Source: CAD feature listing. Evaluate the final solid. Frame: model axes, mm. A direction names the side the tool comes from. Give positions to 0.01 mm unless a question says otherwise; leave off trailing zeros. Write each loop counter-clockwise with the first axis right and the second up, starting at its lowest first coordinate (ties: lowest second). Pieces come first, ordered by that corner, then holes. Notation, with made-up numbers: M 39.5,47 L 60.5,47 A29 cw 60.5,67 Z; hole C -11.75,72 d7. An arc over 180 degrees is marked long. Use CSV: the item, a comma, the result in double quotes. Start each with the question number.
from build123d import *

# Parameters (mm, degrees)
SKETCH1_W               = 15.875
SKETCH1_H               = 15.875
BOSS_EXTRUDE1_DEPTH     = 149.225
CUT_EXTRUDE1_DEPTH      = 151.276811772
CUT_EXTRUDE1_DEPTH_BACK = 151.276811772
CUT_EXTRUDE2_START      = -1.5875
SKETCH4_W               = 12.7
SKETCH4_H               = 14.2875
CUT_EXTRUDE2_DEPTH      = 149.225
CUT_EXTRUDE4_DEPTH      = 151.276811772
SKETCH6_W               = 6.35
SKETCH6_H               = 1.5875
CUT_EXTRUDE5_DEPTH      = 1.5875
SKETCH7_W               = 1.5875
SKETCH7_H               = 0.910155424
CUT_EXTRUDE6_DEPTH      = 1.5875
SKETCH8_R               = 1.5875
SKETCH8_W               = 1.5875
SKETCH8_H               = 3.96875
CUT_EXTRUDE7_DEPTH      = 151.276811772
SKETCH9_R               = 3.175
CUT_EXTRUDE8_DEPTH      = 151.276811772
BOSS_EXTRUDE2_START     = 0.396875
SKETCH10_R              = 1.5875
BOSS_EXTRUDE2_DEPTH     = 0.396875
SKETCH11_W              = 12.7
SKETCH11_H              = 14.601302857
CUT_EXTRUDE9_DEPTH      = 2.54


with BuildPart() as part:
    # Sketch1 → Boss-Extrude1 (new body)
    with BuildSketch(Plane.XY):
        Rectangle(SKETCH1_W, SKETCH1_H)
    extrude(amount=-BOSS_EXTRUDE1_DEPTH)

    # Sketch2 → Cut-Extrude1 (cut, two sides: drawn at the far end of the back side and taken through both)
    with BuildSketch(Plane(origin=(7.9375, 0, 0), x_dir=(0, 0, -1), z_dir=(1, 0, 0)).offset(-CUT_EXTRUDE1_DEPTH_BACK)):
        with BuildLine():
            Line((149.225, 7.9375), (12.7, 7.9375))
            Line((12.7, 7.9375), (31.483553311, 4.7625))
            Line((31.483553311, 4.7625), (109.68727062, 4.7625))
            Line((109.68727062, 4.7625), (112.817862839, 5.291666667))
            Line((112.817862839, 5.291666667), (119.167862839, 5.291666667))
            Line((119.167862839, 5.291666667), (122.298455057, 4.7625))
            Line((122.298455057, 4.7625), (133.410955057, 4.7625))
            Line((133.410955057, 4.7625), (145.71107606, 1.420918197))
            ThreePointArc((145.71107606, 1.420918197), (148.245868191, -0.282331443), (149.225, -3.175))
            Line((149.225, -3.175), (149.225, 7.9375))
        make_face()
        with BuildLine():
            Line((149.225, -7.9375), (149.225, -3.175))
            ThreePointArc((149.225, -3.175), (147.830096045, -6.542596045), (144.4625, -7.9375))
            Line((144.4625, -7.9375), (149.225, -7.9375))
        make_face()
    extrude(amount=CUT_EXTRUDE1_DEPTH + CUT_EXTRUDE1_DEPTH_BACK, mode=Mode.SUBTRACT)

    # Sketch4 → Cut-Extrude2 (cut)
    with BuildSketch(Plane.XY.offset(CUT_EXTRUDE2_START)):
        with Locations((0, 0.79375)):
            Rectangle(SKETCH4_W, SKETCH4_H)
    extrude(amount=-CUT_EXTRUDE2_DEPTH, mode=Mode.SUBTRACT)

    # Sketch5 → Cut-Extrude4 (cut, through all)
    with BuildSketch(Plane.XZ.offset(7.9375)):
        Polygon((2.38125, -6.35), (-2.38125, -6.35), (-4.283584011, -2.497655424), (-6.35, -2.497655424), (-6.35, -1.5875), (-0.79375, -1.5875), (-0.79375, 0), (0.79375, 0), (0.79375, -1.5875), (6.35, -1.5875), (6.35, -2.497655424), (4.283584011, -2.497655424), align=None)
    extrude(amount=-CUT_EXTRUDE4_DEPTH, mode=Mode.SUBTRACT)

    # Sketch6 → Cut-Extrude5 (cut)
    with BuildSketch(Plane.XY):
        Polygon((0.79375, 4.7625), (2.38125, 4.7625), (4.7625, 7.9375), (0.79375, 7.9375), align=None)
        Polygon((-0.79375, 4.7625), (-2.38125, 4.7625), (-4.7625, 7.9375), (-0.79375, 7.9375), align=None)
        with Locations((0, -7.14375)):
            Rectangle(SKETCH6_W, SKETCH6_H)
    extrude(amount=-CUT_EXTRUDE5_DEPTH, mode=Mode.SUBTRACT)

    # Sketch7 → Cut-Extrude6 (cut)
    with BuildSketch(Plane.XZ.offset(7.9375)):
        with Locations((7.14375, -2.042577712)):
            Rectangle(SKETCH7_W, SKETCH7_H)
        with Locations((-7.14375, -2.042577712)):
            Rectangle(SKETCH7_W, SKETCH7_H)
    extrude(amount=-CUT_EXTRUDE6_DEPTH, mode=Mode.SUBTRACT)

    # Sketch8 → Cut-Extrude7 (cut, through all)
    with BuildSketch(Plane(origin=(7.9375, 0, 0), x_dir=(0, 0, -1), z_dir=(1, 0, 0))):
        with Locations((144.4625, -3.175)):
            Circle(SKETCH8_R)
        with Locations((2.38125, -1.190625)):
            Rectangle(SKETCH8_W, SKETCH8_H)
        with BuildLine():
            Line((7.14375, -3.175), (10.31875, -3.175))
            ThreePointArc((10.31875, -3.175), (11.1125, -3.96875), (10.31875, -4.7625))
            Line((10.31875, -4.7625), (7.14375, -4.7625))
            ThreePointArc((7.14375, -4.7625), (6.35, -3.96875), (7.14375, -3.175))
        make_face()
    extrude(amount=-CUT_EXTRUDE7_DEPTH, mode=Mode.SUBTRACT)

    # Sketch9 → Cut-Extrude8 (cut, through all)
    with BuildSketch(Plane.XZ.offset(7.9375)):
        with Locations(Location((0, -22.225, 0), (0, 0, 270))):
            Circle(SKETCH9_R)
        with Locations(Location((0, -122.2375, 0), (0, 0, 270))):
            Circle(SKETCH9_R)
    extrude(amount=-CUT_EXTRUDE8_DEPTH, mode=Mode.SUBTRACT)

    # Sketch10 → Boss-Extrude2 (add)
    with BuildSketch(Plane(origin=(7.9375, 0, 0), x_dir=(0, 0, -1), z_dir=(1, 0, 0)).offset(BOSS_EXTRUDE2_START)):
        with BuildLine():
            Line((144.4625, 0), (19.05, 0))
            ThreePointArc((19.05, 0), (18.25625, -0.79375), (19.05, -1.5875))
            Line((19.05, -1.5875), (141.712869343, -1.5875))
            ThreePointArc((141.712869343, -1.5875), (146.05, -5.924630657), (144.4625, 0))
        make_face()
        with Locations((144.4625, -3.175)):
            Circle(SKETCH10_R, mode=Mode.SUBTRACT)
    boss_extrude2 = extrude(amount=-BOSS_EXTRUDE2_DEPTH)

    # Mirror1: Boss-Extrude2 across plane
    add(boss_extrude2.mirror(Plane(origin=(0, 0, 0), x_dir=(0, 0, 1), z_dir=(1, 0, 0))))

    # Sketch11 → Cut-Extrude9 (cut)
    with BuildSketch(Plane(origin=(0, -6.35, 0), x_dir=(1, 0, 0), z_dir=(0, 1, 0))):
        with Locations((0, 140.711606485)):
            Rectangle(SKETCH11_W, SKETCH11_H)
    extrude(amount=-CUT_EXTRUDE9_DEPTH, mode=Mode.SUBTRACT)


solid = part.part
1. First-contact query: pin 1 (8 mm diameter, centred on x = -2, z = -58, fed in from +Y); pin 2 (3 mm diameter, centred on x = 6.5, y = 2.5, fed in from -Z); pin 3 (0.8 mm diameter, centred on y = -3, z = -1, fed in from -X); pin 4 (4 mm diameter, centred on x = 0, z = -122.24, fed in from -Y). Flat tips, straight axial feed; report the tip coordinate or a pass-through.
2. Access query for faces 1 (the flat face through (-6.35, 0, -74)), 2 (the flat face through (-3.555, 6.328, -0.783)), 3 (the cylindrical face through (0.954, -7.155, -25.253)). Directions: +Z, -Z, +X, -X, +Y, -Y. A direction counts if a zero-diameter tool reaches every point of the face in a straight line with its end or side. Return the directions, or none.
3. Pull-direction query (Z, two-part tool) for faces 4 (the flat face through (8.334, -1, -83)), 5 (the cylindrical face through (0.954, -7.155, -125.266)), 6 (the flat face through (-7.155, 3.115, -139.475)); classes: released by +Z, released by -Z, zero draft, split by the parting line, or undercut.
4. Section C-C on z = -59. Return loops of the section in (x, y).
5. Line query: probe 1 along X at (y, z) = (-5.25, -57.5); probe 2 along Y at (x, z) = (2, -13). Output: solid intervals per line, ascending.
6. Section A-A on z = -9. Give the number of separate pieces and of enclosed holes in the cut face, then the cut area to 3 significant figures.
7. Section B-B on z = -137.5. Return loops of the section in (x, y), then the cut area to 3 significant figures.
Resolved:
1,pin 1,"stops at y = -6.35"
1,pin 2,"stops at z = -146.75"
1,pin 3,"stops at x = -7.94"
1,pin 4,"passes through"
2,face 1,"-Z, +Y"
2,face 2,"+Z, -Z, +Y"
2,face 3,"+Y, -Y"
3,face 4,"zero draft"
3,face 5,"undercut"
3,face 6,"released by -Z"
4,outline,"M -8.33,-1.59 L -7.94,-1.59 L -7.94,-7.94 L 7.94,-7.94 L 7.94,-1.59 L 8.33,-1.59 L 8.33,0 L 7.94,0 L 7.94,4.76 L 6.35,4.76 L 6.35,-6.35 L -6.35,-6.35 L -6.35,4.76 L -7.94,4.76 L -7.94,0 L -8.33,0 Z"
5,probe 1,"x = -7.94 to -6.35, 6.35 to 7.94"
5,probe 2,"y = -7.94 to -6.35"
6,separate pieces,"3"
6,enclosed holes,"0"
6,area,"65.5 mm2"
7,outline,"M -8.33,-1.59 L -7.94,-1.59 L -7.94,-7.94 L -6.35,-7.94 L -6.35,3.65 L -7.94,3.65 L -7.94,0 L -8.33,0 Z; M 6.35,-7.94 L 7.94,-7.94 L 7.94,-1.59 L 8.33,-1.59 L 8.33,0 L 7.94,0 L 7.94,3.65 L 6.35,3.65 Z"
7,area,"38.1 mm2"
